Verification items for the finished model (mm, model axes). A direction names the side the tool comes from. Round coordinates to 2 decimals unless told otherwise and drop trailing zeros. Order: outer loops, then holes, each group sorted by start corner. A loop starts at its lowest first (then second) coordinate and runs counter-clockwise, first axis right, second up. Notation, with made-up numbers: (-23, -28) -> (14, -28) arc R8 ccw to (14, -21) -> close; hole circle Ø9 at (41.5, 4). An arc over 180 degrees is marked (long way). Put each result on its own line as item: value.
```python
from build123d import *

# Parameters (mm, degrees)
BOSS_EXTRUDE1_DEPTH = 6.35
SKETCH2_W           = 20
SKETCH2_H           = 2.5
BOSS_EXTRUDE2_DEPTH = 6.35
SKETCH4_W           = 7
SKETCH4_H           = 2.3
BOSS_EXTRUDE3_DEPTH = 6.35


with BuildPart() as part:
    # Sketch1 → Boss-Extrude1 (new body)
    with BuildSketch(Plane.XY):
        Polygon((-15.235299292, 17.883619427), (-15.235299292, 2.883619427), (-0.235299292, 2.883619427), (-0.235299292, 17.883619427), (2.264700708, 17.883619427), (2.264700708, 0.383619427), (-17.735299292, 0.383619427), (-17.735299292, 17.883619427), align=None)
    extrude(amount=BOSS_EXTRUDE1_DEPTH)

    # Sketch2 → Boss-Extrude2 (add, through all)
    with BuildSketch(Plane.XY):
        with Locations((-7.735299292, 19.133619427)):
            Rectangle(SKETCH2_W, SKETCH2_H)
    extrude(amount=BOSS_EXTRUDE2_DEPTH)

    # Sketch4 → Boss-Extrude3 (add)
    with BuildSketch(Plane.XY.offset(6.35)):
        Polygon((-17.735299292, 20.383619427), (2.264700708, 20.383619427), (2.264700708, 24.083619427), (-4.235299292, 24.083619427), (-4.235299292, 26.383619427), (-11.235299292, 26.383619427), (-11.235299292, 24.083619427), (-17.735299292, 24.083619427), align=None)
        with Locations((-7.735299292, -0.766380573)):
            Rectangle(SKETCH4_W, SKETCH4_H)
    extrude(amount=-BOSS_EXTRUDE3_DEPTH)


solid = part.part
```
Item 1: Sectioned sample at D-D, the plane x = -15.75. Record the boundary of the cut face in (y, z), then the cut area to 3 significant figures.
Geometry check:
outline: (0.38, 0) -> (24.08, 0) -> (24.08, 6.35) -> (0.38, 6.35) -> close
area: 150 mm2
Item 2: Sectioned sample at B-B, the plane z = 3.5. Record the boundary of the cut face in (x, y).
Geometry check:
outline: (-17.74, 0.38) -> (-11.24, 0.38) -> (-11.24, -1.92) -> (-4.24, -1.92) -> (-4.24, 0.38) -> (2.26, 0.38) -> (2.26, 24.08) -> (-4.24, 24.08) -> (-4.24, 26.38) -> (-11.24, 26.38) -> (-11.24, 24.08) -> (-17.74, 24.08) -> close; hole (-15.24, 2.88) -> (-0.24, 2.88) -> (-0.24, 17.88) -> (-15.24, 17.88) -> close
Item 3: Release check for a two-part mould opening along X. For faces 1 (the face through (-1, 0.384, 3)), 2 (the face through (2.265, 12, 3)), 3 (the face through (-8, 2.884, 3)) record: pulls with the +X half, pulls with the -X half, needs draft (parallel to the pull), parting line crosses it, or undercut.
Geometry check:
face 1: needs draft
face 2: pulls with the +X half
face 3: undercut
Item 4: Sectioned sample at A-A, the plane y = 6.25. Record the boundary of the cut face in (x, z), then the cut area to 4 significant figures.
Geometry check:
outline: (-17.74, 0) -> (-15.24, 0) -> (-15.24, 6.35) -> (-17.74, 6.35) -> close; (-0.24, 0) -> (2.26, 0) -> (2.26, 6.35) -> (-0.24, 6.35) -> close
area: 31.75 mm2
Item 5: Material ranges on line 1 along Y through (x, z) = (-1.5, 2.25); line 2 along Y through (x, z) = (-10.5, 1); line 3 along X through (y, z) = (9.5, 4.75), recorded low to high.
Geometry check:
line 1: 0.38 to 2.88, 17.88 to 24.08
line 2: -1.92 to 2.88, 17.88 to 26.38
line 3: -17.74 to -15.24, -0.24 to 2.26
Item 6: Tool access check on faces 4 (the face through (-11.235, 25, 3)), 5 (the face through (-11.235, -1, 3)), 6 (the face through (-15.235, 10, 3)). Record the directions out of +Z, -Z, +X, -X, +Y, -Y that give a thin tool (end or side, any length) a straight path to the whole face; none if there is none.
Geometry check:
face 4: +Z, -Z, -X, +Y
face 5: +Z, -Z, -X, -Y
face 6: +Z, -Z
Item 7: Depth check by flat-ended pin: pin 1 Ø1.8 at (y, z) = (-1, 2.5) entering from -X; pin 2 Ø3 at (x, z) = (-2, 2.5) entering from -Y; pin 3 Ø0.7 at (y, z) = (25.5, 1.5) entering from +X. Enter the tip coordinate at first touch or a pass-through.
Geometry check:
pin 1: x = -11.24
pin 2: y = 0.38
pin 3: x = -4.24
Item 8: Sectioned sample at C-C, the plane x = -10. Record the boundary of the cut face in (y, z).
Geometry check:
outline: (-1.92, 0) -> (2.88, 0) -> (2.88, 6.35) -> (-1.92, 6.35) -> close; (17.88, 0) -> (26.38, 0) -> (26.38, 6.35) -> (17.88, 6.35) -> close
